Print and shaded views of the part. All mm, measured from the part's lowest x, y and z. Coordinates: 2 decimals unless noted, no trailing zeros. Order: outer loops, then holes, each group sorted by start corner. A loop starts at its lowest first (then second) coordinate and runs counter-clockwise, first axis right, second up.
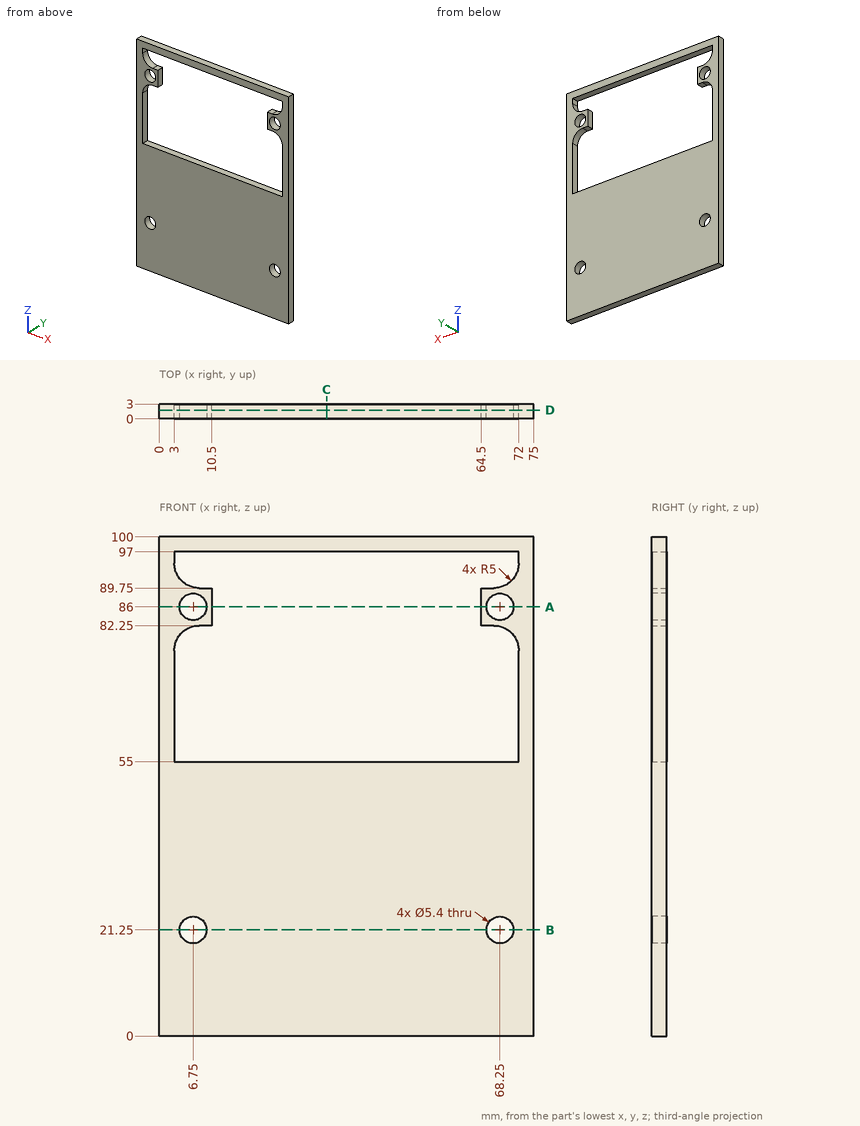
Q1. Cut at B-B, the plane z = 21.25. List the corners of the cut face in (x, y).
Established:
outline: (0, 0) - (4.05, 0) - (4.05, 3) - (0, 3) - close; (9.45, 0) - (65.55, 0) - (65.55, 3) - (9.45, 3) - close; (70.95, 0) - (75, 0) - (75, 3) - (70.95, 3) - close
Q2. Cut at A-A, the plane z = 86. List the corners of the cut face in (x, y), plus the area to 3 significant figures.
Established:
outline: (0, 0) - (4.05, 0) - (4.05, 3) - (0, 3) - close; (9.45, 0) - (10.5, 0) - (10.5, 3) - (9.45, 3) - close; (64.5, 0) - (65.55, 0) - (65.55, 3) - (64.5, 3) - close; (70.95, 0) - (75, 0) - (75, 3) - (70.95, 3) - close
area: 30.6 mm2
Q3. Cut at C-C, the plane x = 33.5. List the corners of the cut face in (y, z), plus the area to 3 significant figures.
Established:
outline: (0, 0) - (3, 0) - (3, 55) - (0, 55) - close; (0, 97) - (3, 97) - (3, 100) - (0, 100) - close
area: 174 mm2
Q4. Cut at D-D, the plane y = 1.75. List the corners of the cut face in (x, z), plus the area to 3 significant figures.
Established:
outline: (0, 0) - (75, 0) - (75, 100) - (0, 100) - close; hole (3, 55) - (72, 55) - (72, 77.25) arc R5 ccw to (67, 82.25) - (64.5, 82.25) - (64.5, 89.75) - (67, 89.75) arc R5 ccw to (72, 94.75) - (72, 97) - (3, 97) - (3, 94.75) arc R5 ccw to (8, 89.75) - (10.5, 89.75) - (10.5, 82.25) - (8, 82.25) arc R5 ccw to (3, 77.25) - close; hole circle Ø5.4 at (6.75, 21.25); hole circle Ø5.4 at (6.75, 86); hole circle Ø5.4 at (68.25, 21.25); hole circle Ø5.4 at (68.25, 86)
area: 4,640 mm2
Q5. Probe line 1 (Z direction, x = 36.5, y = 0.8); line 2 (X direction, y = 2.3, z = 71); line 3 (Z direction, x = 6.75, y = 2.45). List the from-to ranges inside material, lowest first.
Established:
line 1: z = 0 to 55, 97 to 100
line 2: x = 0 to 3, 72 to 75
line 3: z = 0 to 18.55, 23.95 to 55, 82.09 to 83.3, 88.7 to 89.91, 97 to 100
